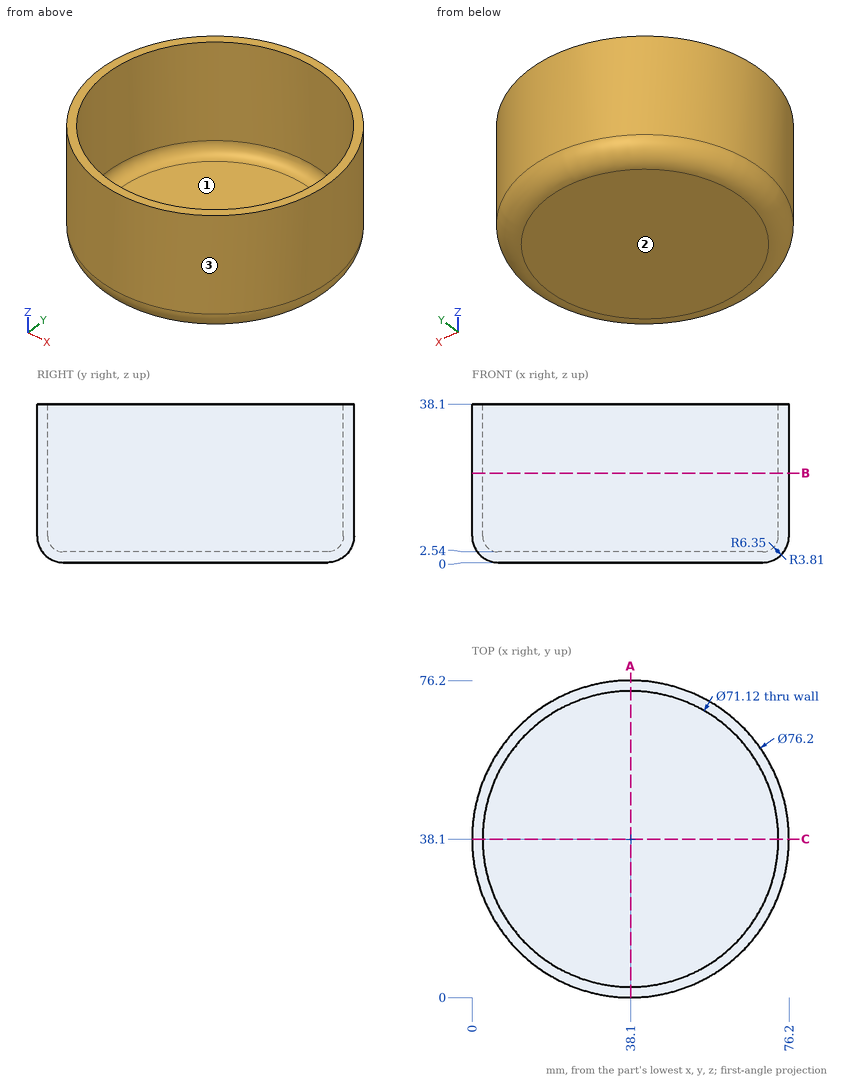
Verification items for this drawing (mm, ordinates from the low corner). Round coordinates to 2 decimals unless told otherwise and drop trailing zeros. Order: outer loops, then holes, each group sorted by start corner. A loop starts at its lowest first (then second) coordinate and runs counter-clockwise, first axis right, second up. Notation, with made-up numbers: (62.5, 23) - (116.5, 23) arc R11 cw to (116.5, 30) - close; hole circle Ø10 at (45.5, -38). An arc over 180 degrees is marked (long way). Use CSV: the item, a comma, the result in double quotes.
(1) Thickness scan on probe 1 along Y at (x, z) = (38.1, 27); probe 2 along Z at (x, y) = (66, 39.5); probe 3 along Z at (x, y) = (8, 27). Record the ranges inside material, lowest first. Write a range as from..to.
Entries:
probe 1,"0..2.54, 73.66..76.2"
probe 2,"0..2.54"
probe 3,"0.01..2.55"
(2) Section check A-A on x = 38.1. Record the boundary of the cut face in (y, z), and give its area (3 significant figures).
Entries:
outline,"(0, 6.35) arc R6.35 ccw to (6.35, 0) - (69.85, 0) arc R6.35 ccw to (76.2, 6.35) - (76.2, 38.1) - (73.66, 38.1) - (73.66, 6.35) arc R3.81 cw to (69.85, 2.54) - (6.35, 2.54) arc R3.81 cw to (2.54, 6.35) - (2.54, 38.1) - (0, 38.1) - close"
area,"363 mm^2"
(3) Gauge pin test, flat ends, axial feed: pin 1 Ø2 at (x, z) = (26, 10.5) entering from +Y; pin 2 Ø2 at (y, z) = (44, 34) entering from -X; pin 3 Ø1.5 at (y, z) = (33.5, 21.5) entering from -X (3 decimals). Record the tip position at first contact, or that the pin passes through.
Entries:
pin 1,"y = 74.55"
pin 2,"x = 0.32"
pin 3,"x = 0.195"
(4) Mould release check, pull along Y, two halves, no side actions. Record for the marked faces 1, 2 and 3: released by +Y, released by -Y, zero draft, split by the parting line, or undercut.
Entries:
face 1,"undercut"
face 2,"zero draft"
face 3,"split by the parting line"
(5) Section check B-B on z = 21.5. Record the boundary of the cut face in (x, y).
Entries:
outline,"circle Ø76.2 at (38.1, 38.1); hole circle Ø71.12 at (38.1, 38.1)"
